Read the model definition and answer for the solid it produces. Units are mm, in the model's axes. A direction names the side the tool comes from. Round coordinates to 2 decimals unless told otherwise and drop trailing zeros. Write each loop counter-clockwise with the first axis right and the second up, starting at its lowest first coordinate (ties: lowest second). Pieces come first, ordered by that corner, then holes. Notation, with made-up numbers: (60, 50.5) - (106, 50.5) arc R23 ccw to (106, 72.5) - close; hole circle Ø9 at (-33.5, 48). An arc over 180 degrees is marked (long way). Answer as CSV lines item,"result". Start each with the question number.
1) Consider line 1 along Y through (x, z) = (-308.5, -95); line 2 along X through (y, z) = (-512, 95); line 3 along Y through (x, z) = (319.5, -103). Determine where each line is inside the solid, lowest interval first.
2) Which of the six approach directions +Z, -Z, +X, -X, +Y, -Y give full straight-line access (tool end or side, diameter ignored) to faces 4 (the flat face through (474, -506, -1)), 5 (the flat face through (-300, 437, 71)), 6 (the cylindrical face through (-308.11, 443.43, 107.3)), 7 (the cylindrical face through (289.57, -508.11, 107.3)), 8 (the flat face through (135, 104, 95))?
3) Find section B-B on x = 419. Determine the outline of the cut face in (y, z) (1 decimal).
4) Find section D-D on y = -292. Determine the outline of the cut face in (x, z).
5) For a pull along Y with two mould halves and no side action, classify faces 1 (the flat face through (-100, -158.9, 1.3)), 2 (the cylindrical face through (-308.11, 649.13, 98.36)), 3 (the cylindrical face through (163.87, -508.11, 98.36)) as +Y half, -Y half, draft (parallel to the pull), parting line (faces both ways), or undercut.
6) Find section C-C on x = 34.5. Determine the outline of the cut face in (y, z).
7) Find section A-A on y = 634. Determine the outline of the cut face in (x, z), then the cut area to 3 significant figures.
8) Each of these flat-tipped pins is pushed along its axis until it touches: pin 1 (1.5 mm diameter, centred on x = 16.5, z = -91, fed in from +Y); pin 2 (12 mm diameter, centred on x = 286.5, z = -43.5, fed in from +Y); pin 3 (1.5 mm diameter, centred on x = -106, z = -5.5, fed in from -Y). Where does it stop, or does it pass through?
from build123d import *

# Parameters (mm, degrees)
SKETCH_1_W          = 774
SKETCH_1_H          = 1179
EXTRUDE_1_DEPTH     = 4
CUT_EXTRUDE_2_DEPTH = 8
SKETCH_3_W          = 280
SKETCH_3_H          = 490
EXTRUDE_3_DEPTH     = 16
SKETCH_4_R          = 15.5
CUT_EXTRUDE_4_DEPTH = 16
EXTRUDE_5_DEPTH     = 12
SKETCH_7_W          = 350
SKETCH_7_H          = 280
EXTRUDE_6_DEPTH     = 16
SKETCH_8_R          = 15.5
CUT_EXTRUDE_7_DEPTH = 16
SKETCH_9_W          = 190
SKETCH_9_H          = 1300
EXTRUDE_8_DEPTH     = 12


with BuildPart() as part:
    # 草图1 → 拉伸1 (new, symmetric)
    with BuildSketch(Plane.XY):
        with Locations((87, 89.5)):
            Rectangle(SKETCH_1_W, SKETCH_1_H)
    extrude(amount=EXTRUDE_1_DEPTH, both=True)

    # 草图2 → 拉伸2 (cut)
    with BuildSketch(Plane.XY.offset(4)):
        Polygon((-300, -500), (-300, 189), (124, -500), align=None)
        Polygon((-226, 679), (474, -458.5), (474, 679), align=None)
    extrude(amount=-CUT_EXTRUDE_2_DEPTH, mode=Mode.SUBTRACT)

    # 草图3 → 拉伸3 (add)
    with BuildSketch(Plane.ZY.offset(300)):
        with Locations((0, 434)):
            Rectangle(SKETCH_3_W, SKETCH_3_H)
    extrude(amount=EXTRUDE_3_DEPTH)

    # 草图4 → 拉伸4 (cut)
    with BuildSketch(Plane.ZY.offset(316)):
        with Locations((-95, 634)):
            Circle(SKETCH_4_R)
        with Locations((-95, 434)):
            Circle(SKETCH_4_R)
        with Locations((-95, 234)):
            Circle(SKETCH_4_R)
        with Locations(Location((95, 234, 0), (0, 0, 180))):
            Circle(SKETCH_4_R)
        with Locations(Location((95, 434, 0), (0, 0, 180))):
            Circle(SKETCH_4_R)
        with Locations(Location((95, 634, 0), (0, 0, 180))):
            Circle(SKETCH_4_R)
    extrude(amount=-CUT_EXTRUDE_4_DEPTH, mode=Mode.SUBTRACT)

    # 草图5 → 拉伸5 (add)
    with BuildSketch(Plane(origin=(-133.236051502, -81.991416309, 0), x_dir=(0, 0, 1), z_dir=(-0.8516583167045437, -0.5240974256643349, 0))):
        Polygon((0, 306.578208367), (95, 306.578208367), (95, -483.421791633), (-95, -483.421791633), (-95, 306.578208367), align=None)
    extrude(amount=EXTRUDE_5_DEPTH)

    # 草图7 → 拉伸6 (add)
    with BuildSketch(Plane.XZ.offset(500)):
        with Locations((299, 0)):
            Rectangle(SKETCH_7_W, SKETCH_7_H)
    extrude(amount=EXTRUDE_6_DEPTH)

    # 草图8 → 拉伸7 (cut)
    with BuildSketch(Plane.XZ.offset(516)):
        with Locations(Location((179, 95, 0), (0, 0, 270))):
            Circle(SKETCH_8_R)
        with Locations(Location((299, 95, 0), (0, 0, 270))):
            Circle(SKETCH_8_R)
        with Locations(Location((419, 95, 0), (0, 0, 270))):
            Circle(SKETCH_8_R)
        with Locations(Location((419, -95, 0), (0, 0, 90))):
            Circle(SKETCH_8_R)
        with Locations(Location((299, -95, 0), (0, 0, 90))):
            Circle(SKETCH_8_R)
        with Locations(Location((179, -95, 0), (0, 0, 90))):
            Circle(SKETCH_8_R)
    extrude(amount=-CUT_EXTRUDE_7_DEPTH, mode=Mode.SUBTRACT)

    # 草图9 → 拉伸8 (add)
    with BuildSketch(Plane(origin=(139.150214592, 85.630901288, 0), x_dir=(0, 0, -1), z_dir=(0.8516583167045437, 0.5240974256643349, 0))):
        with Locations((0, 26.722015243)):
            Rectangle(SKETCH_9_W, SKETCH_9_H)
    extrude(amount=EXTRUDE_8_DEPTH)


solid = part.part
Check values:
1,line 1,"y = 189 to 218.5, 249.5 to 418.5, 449.5 to 618.5, 649.5 to 679"
1,line 2,"x = 124 to 163.5, 194.5 to 283.5, 314.5 to 403.5, 434.5 to 474"
1,line 3,"y = -516 to -500"
2,face 4,"+Z, -Z, +X, -Y"
2,face 5,"+Z, +Y"
2,face 6,"-X"
2,face 7,"-Y"
2,face 8,"+Z, +X, +Y"
3,outline,"(-516, -140) - (-500, -140) - (-500, -110.5) - (-516, -110.5) - close; (-516, -79.5) - (-500, -79.5) - (-500, -4) - (-369.1, -4) - (-369.1, -95) - (-346.2, -95) - (-346.2, 95) - (-369.1, 95) - (-369.1, 4) - (-500, 4) - (-500, 79.5) - (-516, 79.5) - close; (-516, 110.5) - (-500, 110.5) - (-500, 140) - (-516, 140) - close"
4,outline,"(-18.09, -95) - (-4, -95) - (-4, -4) - (371.54, -4) - (371.54, -95) - (385.63, -95) - (385.63, 95) - (371.54, 95) - (371.54, 4) - (-4, 4) - (-4, 95) - (-18.09, 95) - close"
5,face 1,"-Y half"
5,face 2,"undercut"
5,face 3,"draft"
6,outline,"(-377.46, -95) - (-354.56, -95) - (-354.56, -4) - (255.69, -4) - (255.69, -95) - (278.58, -95) - (278.58, 95) - (255.69, 95) - (255.69, 4) - (-354.56, 4) - (-354.56, 95) - (-377.46, 95) - close"
7,outline,"(-316, -140) - (-300, -140) - (-300, -110.5) - (-316, -110.5) - close; (-316, -79.5) - (-300, -79.5) - (-300, -4) - (-198.31, -4) - (-198.31, -95) - (-184.22, -95) - (-184.22, 95) - (-198.31, 95) - (-198.31, 4) - (-300, 4) - (-300, 79.5) - (-316, 79.5) - close; (-316, 110.5) - (-300, 110.5) - (-300, 140) - (-316, 140) - close"
7,area,"6,980 mm^2"
8,pin 1,"stops at y = 309.05"
8,pin 2,"stops at y = -121.17"
8,pin 3,"stops at y = -150.37"
